Geometry check sheet. Reference: the model listing, model coordinates, mm. Face numbers are marked on the shaded views. A direction names the side the tool comes from. Round coordinates to 2 decimals unless told otherwise and drop trailing zeros. Loops run counter-clockwise (first coordinate to the right, second up) from the corner with the lowest first, then second, coordinate; pieces in that order, holes last. Notation, with made-up numbers: (82.25, -23) -> (113.25, -23) arc R30 ccw to (113.25, 5) -> close; hole circle Ø4 at (18, -26). An arc over 180 degrees is marked (long way). Use one line per item in the form item = value.
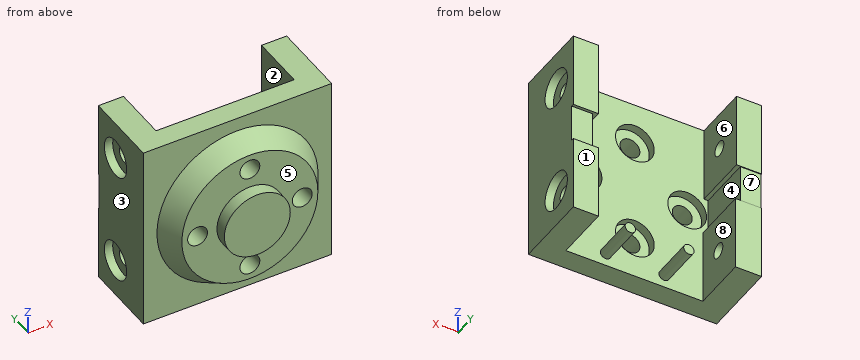
Autodesk Inventor part; units mm, degrees
ref_plane "YZ Plane" through (0, 0, 0) normal (1, 0, 0) x (0, 1, 0)
ref_plane "XZ Plane" through (0, 0, 0) normal (0, 1, 0) x (-1, 0, 0)
ref_plane "XY Plane" through (0, 0, 0) normal (0, 0, 1) x (1, 0, 0)
sketch "Szkic1" plane through (0, 0, 0) normal (0, 1, 0) x (-1, 0, 0)
  circle A0 centre (0, 0) radius 32.5
  dimension "d0" = 65
extrude "Wyciągnięcie proste1" add sketch "Szkic1" along normal blind 10
sketch "Szkic2" plane through (0, 10, 0) normal (0, 1, 0) x (1, 0, 0)
  circle A0 centre (0, 0) radius 15.75
  circle A1 centre (0, 25) radius 4.75
  circle A2 centre (-25, 0) radius 4.75
  circle A3 centre (0, -25) radius 4.75
  circle A4 centre (25, 0) radius 4.75
  dimension "d3" = 31.5
  dimension "d4" = 9.5
  dimension "d5" = 25
  dimension "d8" = 360
extrude "Wyciągnięcie proste2" cut sketch "Szkic2" against normal blind 23.25 contours A1 | A2 | A3 | A4
sketch "Szkic3" plane through (0, 0, 0) normal (0, -1, 0) x (1, 0, 0)
  circle A0 centre (0, 0) radius 15.75
  dimension "d12" = 31.5
extrude "Wyciągnięcie proste3" add sketch "Szkic3" along normal blind 6
sketch "Szkic4" plane through (0, 10, 0) normal (0, 1, 0) x (1, 0, 0)
  line L0 (-45, 45) -> (45, 45)
  line L1 (45, 45) -> (45, -45)
  line L2 (45, -45) -> (-45, -45)
  line L3 (-45, -45) -> (-45, 45)
  point P0 (0, 0)
  point P1 (0, 45)
  point P2 (45, 0)
  dimension "d15" = 90
  dimension "d16" = 90
extrude "Wyciągnięcie proste4" add sketch "Szkic4" along normal blind 10
sketch "Szkic5" plane through (0, 10, 0) normal (0, -1, 0) x (1, 0, 0)
  circle A0 centre (-25, 0) radius 4.75
  circle A1 centre (0, 25) radius 4.75
  circle A2 centre (25, 0) radius 4.75
  circle A3 centre (0, -25) radius 4.75
  point P0 (0, 0)
extrude "Wyciągnięcie proste5" cut sketch "Szkic5" along normal mid plane 50
sketch "Szkic6" plane through (0, 20, 0) normal (0, 1, 0) x (1, 0, 0)
  circle A0 centre (0, 25) radius 4.75
  circle A1 centre (25, 0) radius 4.75
  circle A2 centre (-25, 0) radius 4.75
  circle A3 centre (0, -25) radius 4.75
  circle A4 centre (-25, 0) radius 9.25
  circle A5 centre (0, 0) radius 15.75
  circle A6 centre (0, 25) radius 9.25
  circle A7 centre (25, 0) radius 4.75
  circle A8 centre (25, 0) radius 9.25
  circle A9 centre (0, -25) radius 9.25
extrude "Wyciągnięcie proste6" cut sketch "Szkic6" against normal blind 4 contours A4 | A6 | A8 | A9
sketch "Szkic7" plane through (0, 10, 0) normal (0, -1, 0) x (1, 0, 0)
  circle A0 centre (0, 0) radius 38.5
  dimension "d29" = 77
sketch "Szkic8" plane through (0, 0, 0) normal (0, -1, 0) x (1, 0, 0)
  circle A0 centre (0, 0) radius 32.5
loft "Wyciągnięcie złożone1" add profiles "Szkic7" section 2 edges at (32.5, 0, 0)
sketch "Szkic9" plane through (0, 0, 0) normal (0, -1, 0) x (1, 0, 0)
  circle A0 centre (0, -25) radius 4.75
  circle A1 centre (-25, 0) radius 4.75
  circle A2 centre (0, 25) radius 4.75
  circle A3 centre (25, 0) radius 4.75
  point P0 (0, 0)
extrude "Wyciągnięcie proste7" cut sketch "Szkic9" against normal blind 30
sketch "Szkic10" plane through (0, 20, 0) normal (0, 1, 0) x (1, 0, 0)
  line L0 (-45, -45) -> (-45, 45)
  line L1 (-45, -45) -> (-33, -45)
  line L2 (-33, -45) -> (-33, -9)
  line L3 (-33, -9) -> (-45, -9)
  line L4 (-45, -9) -> (-45, -45)
  line L5 (-45, 45) -> (-32.5, 45)
  line L6 (-32.5, 45) -> (-32.5, 9)
  line L7 (-32.5, 9) -> (-45, 9)
  line L8 (-45, 9) -> (-45, 45)
  line L9 (45, -45) -> (-45, -45)
  line L10 (45, -45) -> (33, -45)
  line L11 (33, -45) -> (33, -9)
  line L12 (33, -9) -> (45, -9)
  line L13 (45, -9) -> (45, -45)
  line L14 (45, 45) -> (33, 45)
  line L15 (33, 45) -> (33, 9)
  line L16 (33, 9) -> (45, 9)
  line L17 (45, 9) -> (45, 45)
  point P0 (0, 0)
  dimension "d30" = 12
  dimension "d31" = 36
extrude "Wyciągnięcie proste8" add sketch "Szkic10" along normal blind 26.325
sketch "Szkic11" plane through (45, 10, 45) normal (1, 0, 0) x (0, 0, -1)
  circle A0 centre (18, 22.5) radius 5
  circle A1 centre (72, 22.5) radius 5
  point P0 (45, -10)
  dimension "d34" = 10
  dimension "d35" = 10
sketch "Szkic12" plane through (-45, 10, -45) normal (-1, 0, 0) x (0, 0, 1)
  circle A0 centre (18, 22.5) radius 5
  circle A1 centre (72, 22.5) radius 5
  point P0 (45, -10)
  dimension "d36" = 10
  dimension "d37" = 10
sketch "Szkic13" plane through (-45, 10, -45) normal (-1, 0, 0) x (0, 0, 1)
  point P0 (45, -10)
sketch "Szkic14" plane through (-45, 10, -45) normal (-1, 0, 0) x (0, 0, 1)
  line L0 (36, 10) -> (54, 10)
  line L1 (36, 10) -> (54, 10)
  line L2 (54, 10) -> (54, 36)
  line L3 (54, 36) -> (36, 36)
  line L4 (36, 36) -> (36, 10)
  point P0 (45, -10)
extrude "Wyciągnięcie proste9" add sketch "Szkic14" against normal blind 10
sketch "Szkic15" plane through (45, 10, 45) normal (1, 0, 0) x (0, 0, -1)
  line L0 (36, 10) -> (36, 36.325)
  line L1 (54, 10) -> (54, 36.325)
  line L2 (36, 10) -> (54, 10)
  line L3 (54, 10) -> (54, 35)
  line L4 (54, 35) -> (36, 35)
  line L5 (36, 35) -> (36, 10)
  point P0 (45, -10)
extrude "Wyciągnięcie proste10" add sketch "Szkic15" against normal blind 10
hole "Otwór1" at (45, 32.5, 27) at (45, 32.5, -27) direction (-1, 0, 0) diameter 7.188 depth 24 tip angle 118 counterbore diameter 18 counterbore depth 4
hole "Otwór2" at (-45, 32.5, -27) at (-45, 32.5, 27) direction (1, 0, 0) diameter 7.188 depth 20 tip angle 118 counterbore diameter 18 counterbore depth 4
sketch "Szkic16" plane through (0, 20, 0) normal (0, 1, 0) x (1, 0, 0)
  circle A0 centre (14, 39) radius 2.5
  circle A1 centre (-14, 39) radius 2.5
  point P0 (0, 0)
  dimension "d56" = 5
  dimension "d57" = 5
extrude "Wyciągnięcie proste11" add sketch "Szkic16" along normal blind 20
sketch "Szkic17" plane through (0, 20, 0) normal (0, 1, 0) x (1, 0, 0)
  point P0 (0, 0)
properties part number "polaczenie_CH-R"
1. Gauge pin test, flat ends, axial feed: pin 1 (6 mm diameter, centred on y = 34, z = -25, fed in from +X); pin 2 (9 mm diameter, centred on x = -21, z = 2.5, fed in from +Y); pin 3 (9.5 mm diameter, centred on y = 32.5, z = -27, fed in from -X). Record the tip position at first contact, or that the pin passes through.
Return value:
pin_1 = 41
pin_2 = 16
pin_3 = -41
2. Tool access check on the marked faces 4, 5, 6, 7 and 8. Record the directions out of +Z, -Z, +X, -X, +Y, -Y that give a thin tool (end or side, any length) a straight path to the whole face; none if there is none.
Return value:
face_4 = +Y
face_5 = -Y
face_6 = +Z, +Y
face_7 = +X, -X, +Y
face_8 = +Z, -Z, +Y
3. Section check A-A (x = 0). Record the boundary of the cut face in (y, z).
Return value:
outline = (-6, -15.75) -> (0, -15.75) -> (0, -20.25) -> (16, -20.25) -> (16, -15.75) -> (20, -15.75) -> (20, 15.75) -> (16, 15.75) -> (16, 20.25) -> (0, 20.25) -> (0, 15.75) -> (-6, 15.75) -> close; (0, -32.5) -> (10, -38.5) -> (10, -45) -> (20, -45) -> (20, -34.25) -> (16, -34.25) -> (16, -29.75) -> (0, -29.75) -> close; (0, 29.75) -> (16, 29.75) -> (16, 34.25) -> (20, 34.25) -> (20, 45) -> (10, 45) -> (10, 38.5) -> (0, 32.5) -> close
4. Section check C-C (y = 32.5). Count the separate pieces of the cut face and the enclosed holes in it, then the cut area to 3 significant figures.
Return value:
separate_pieces = 8
enclosed_holes = 0
area = 1,620 mm2
5. Mould release check, pull along X, two halves, no side actions. Record for the marked faces 1, 2 and 3: released by +X, released by -X, zero draft, split by the parting line, or undercut.
Return value:
face_1 = zero draft
face_2 = undercut
face_3 = released by -X
6. Material ranges on line 1 along Z through (x, y) = (0, 18.4); line 2 along Z through (x, y) = (39, 32.5); line 3 along X through (y, z) = (30, 12), recorded low to high.
Return value:
line_1 = -45 to -34.25, -15.75 to 15.75, 34.25 to 45
line_2 = -45 to -30.59, -23.41 to 23.41, 30.59 to 45
line_3 = -45 to -33, 33 to 45
7. Section check B-B (y = 3.5). Record the boundary of the cut face in (x, z).
Return value:
outline = circle Ø69.2 at (0, 0); hole circle Ø9.5 at (-25, 0); hole circle Ø9.5 at (0, -25); hole circle Ø9.5 at (0, 25); hole circle Ø9.5 at (25, 0)
